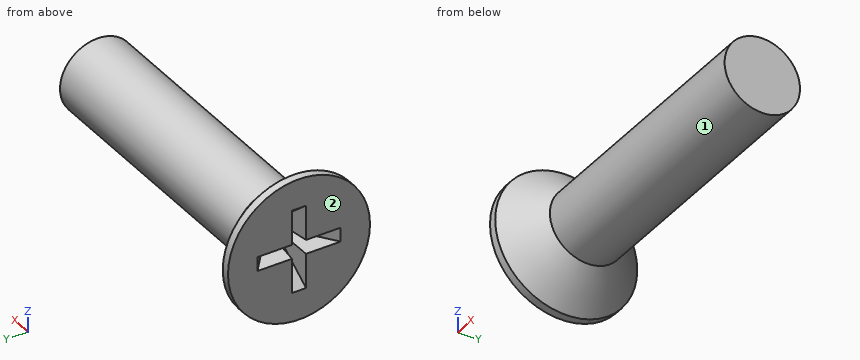
```python
from build123d import *

# Parameters (mm, degrees)
SKETCH3_W         = 1.12
SKETCH3_H         = 6.62
SKETCH4_W         = 0.56
SKETCH4_H         = 0.56
CIRPATTERN1_COUNT = 2
CIRPATTERN1_ANGLE = 90


with BuildPart() as part:
    # BodySke → Base-Revolve (revolve)
    with BuildSketch(Plane.XY):
        Polygon((0, 0), (0, 5.65), (0.65, 5.65), (3.3, 3), (25, 3), (25, 0), align=None)
    revolve(axis=Axis((-6.35, 0, 0), (1, 0, 0)))

    # Sketch3 → Cross section 0
    with BuildSketch(Plane.ZY):
        Rectangle(SKETCH3_W, SKETCH3_H)
    # Sketch4 → Cross section 1
    with BuildSketch(Plane.ZY.offset(-3.61)):
        Rectangle(SKETCH4_W, SKETCH4_H)
    cross = loft(mode=Mode.SUBTRACT)

    # CirPattern1: Cross ×2 about axis
    cirpattern1_axis = Axis((0, 0, 0), (1, 0, 0))
    for i in range(1, CIRPATTERN1_COUNT):
        add(cross.rotate(cirpattern1_axis, i * CIRPATTERN1_ANGLE / (CIRPATTERN1_COUNT - 1)), mode=Mode.SUBTRACT)


solid = part.part
```
Geometry check sheet. Reference: the model listing, model coordinates, mm. Face numbers are marked on the shaded views. A direction names the side the tool comes from. Give positions to 0.01 mm unless a question says otherwise; leave off trailing zeros. Write each loop counter-clockwise with the first axis right and the second up, starting at its lowest first coordinate (ties: lowest second). Pieces come first, ordered by that corner, then holes. Notation, with made-up numbers: (76.25, 53.5) -> (81.25, 53.5) arc R33 ccw to (81.25, 92.5) -> close; hole circle Ø10 at (71.5, -39). An arc over 180 degrees is marked (long way). One line per question, with ' | ' between items.
Item 1: Sectioned sample at A-A, the plane x = 5. Record the boundary of the cut face in (y, z), plus the area to 3 significant figures.
Determined:
outline: circle Ø6 at (0, 0) | area: 28.3 mm^2
Item 2: Scan lines: line 1 along X through (y, z) = (1.5, 4); line 2 along Y through (x, z) = (8.25, 1.5); line 3 along X through (y, z) = (3.75, -0.75). Record each from-to range of solid material in increasing order.
Determined:
line 1: 0 to 2.03 | line 2: -2.6 to 2.6 | line 3: 0 to 2.48
Item 3: Depth check by flat-ended pin: pin 1 (1.5 mm diameter, centred on x = 21.5, z = -3, fed in from -Y); pin 2 (6 mm diameter, centred on x = 6, y = -1.5, fed in from +Z); pin 3 (3 mm diameter, centred on x = 16.5, z = -1, fed in from -Y); pin 4 (6 mm diameter, centred on y = 4, z = 2.5, fed in from +X). Enter the tip coordinate at first touch or a pass-through.
Determined:
pin 1: y = -1.98 | pin 2: z = 3.12 | pin 3: y = -3 | pin 4: x = 25
Item 4: Access from +Z, -Z, +X, -X, +Y, -Y to the whole of each face (thin tool, end or side, straight path). Record for the marked faces 1 and 2.
Determined:
face 1: +X | face 2: +Z, -Z, -X, +Y, -Y
